from build123d import *

# Parameters (mm, degrees)
SKETCH1_W           = 1.524
SKETCH1_H           = 1.524
BOSS_EXTRUDE1_DEPTH = 1.524


with BuildPart() as part:
    # Sketch1 → Boss-Extrude1 (new body)
    with BuildSketch(Plane.XY):
        with BuildLine():
            Line((-22.225726205, -1.524), (-22.225726205, -2.14505284))
            Line((-22.225726205, -2.14505284), (-23.442995373, -2.14505284))
            ThreePointArc((-23.442995373, -2.14505284), (-30.161746406, -5.595987037), (-34.709680239, -11.626481223))
            ThreePointArc((-34.709680239, -11.626481223), (-32.790024922, -0.986396807), (-26.958529189, 8.1180049))
            ThreePointArc((-26.958529189, 8.1180049), (-25.191828644, 9.462219786), (-24.078033866, 7.541905835))
            ThreePointArc((-24.078033866, 7.541905835), (-25.02470469, 4.216402452), (-24.348732091, 0.8255))
            Line((-24.348732091, 0.8255), (-22.225726205, 0.8255))
            Line((-22.225726205, 0.8255), (-22.225726205, -1.524))
        make_face()
        with Locations((-26.716818925, -0.762)):
            Rectangle(SKETCH1_W, SKETCH1_H, mode=Mode.SUBTRACT)
    extrude(amount=BOSS_EXTRUDE1_DEPTH)


solid = part.part
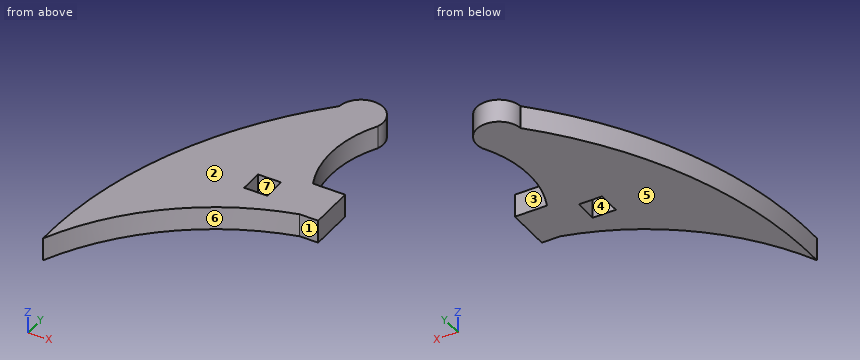
Can you work these out from the model? Positions are in its coordinate system, mm. Face numbers are marked on the shaded views. A direction names the side the tool comes from. Give positions to 0.01 mm unless a question says otherwise; leave off trailing zeros. Loops run counter-clockwise (first coordinate to the right, second up) from the corner with the lowest first, then second, coordinate; pieces in that order, holes last. Notation, with made-up numbers: (-31, -8.75) -> (24, -8.75) arc R10 cw to (24, 6.25) -> close; hole circle Ø9 at (34.5, 72). An arc over 180 degrees is marked (long way). Return JSON: item names as keys, results as strings.
Q1. I want a section at C-C, the plane y = -1.25. List the corners of the cut face in (x, z) for me.
Checks:
{"outline": "(-32.89, 0) -> (-27.48, 0) -> (-27.48, 1.52) -> (-32.89, 1.52) -> close; (-25.95, 0) -> (-22.23, 0) -> (-22.23, 1.52) -> (-25.95, 1.52) -> close"}
Q2. I need wall thicknesses on probe 1 along Y at (x, z) = (-23, 0.65); probe 2 along X at (y, z) = (-1.25, 0.4); probe 3 along X at (y, z) = (-1, 1.1). Which ranges of each line are inside material? Lowest first, please.
Checks:
{"probe 1": "y = -2.15 to 0.83", "probe 2": "x = -32.89 to -27.48, -25.95 to -22.23", "probe 3": "x = -32.8 to -27.48, -25.95 to -22.23"}
Q3. I want a section at D-D, the plane x = -22.75. List the corners of the cut face in (y, z) for me, then the cut area to 3 significant figures.
Checks:
{"outline": "(-2.15, 0) -> (0.83, 0) -> (0.83, 1.52) -> (-2.15, 1.52) -> close", "area": "4.53 mm2"}
Q4. I want a section at A-A, the plane x = -24.75. List the corners of the cut face in (y, z) for me, then the cut area to 3 significant figures.
Checks:
{"outline": "(-2.53, 0) -> (1.91, 0) -> (1.91, 1.52) -> (-2.53, 1.52) -> close; (5.93, 0) -> (9.3, 0) -> (9.3, 1.52) -> (5.93, 1.52) -> close", "area": "11.9 mm2"}
Q5. I want a section at B-B, the plane z = 0.8. List the corners of the cut face in (x, y) for me, then the cut area to 3 significant figures.
Checks:
{"outline": "(-34.71, -11.63) arc R16.92 cw to (-23.44, -2.15) -> (-22.23, -2.15) -> (-22.23, 0.83) -> (-24.35, 0.83) arc R7.36 cw to (-24.08, 7.54) arc R1.48 ccw (long way) to (-26.96, 8.12) arc R27.82 ccw to start; hole (-27.48, -1.52) -> (-25.95, -1.52) -> (-25.95, 0) -> (-27.48, 0) -> close", "area": "101 mm2"}
Q6. On a 3-axis mill with a long thin cutter (end or side, diameter ignored), from which of +Z, -Z, +X, -X, +Y, -Y can I reach the whole of each face in a straight line? I mean the marked faces 1, 2 and 3. Say none if no direction works.
Checks:
{"face 1": "+Z, -Z, +X, -Y", "face 2": "+Z, +X, -X, +Y, -Y", "face 3": "+Z, -Z, +X"}
Q7. We'd pull the mould along Y, two halves only. Please class the marked faces 4, 5, 6 and 7: released by +Y, released by -Y, zero draft, split by the parting line, or undercut.
Checks:
{"face 4": "undercut", "face 5": "zero draft", "face 6": "released by -Y", "face 7": "undercut"}
